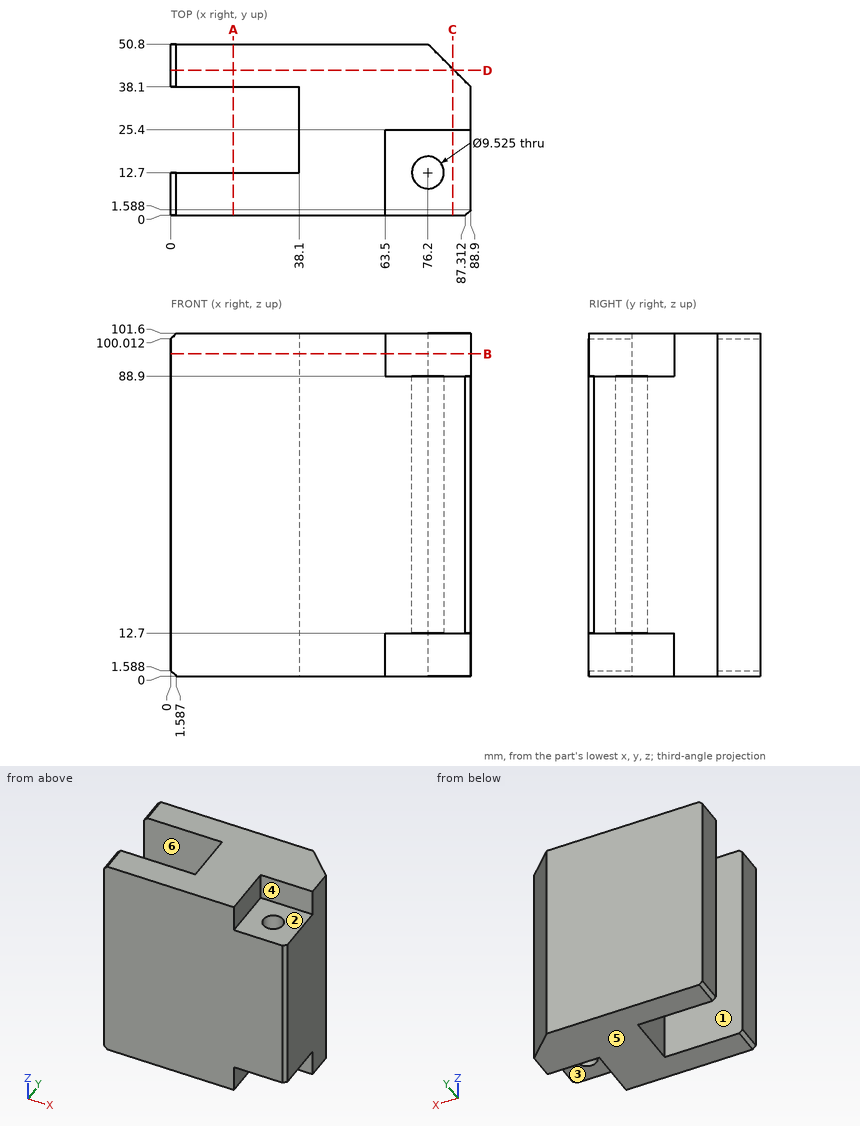
Here's the drawing with two shaded views (mm, measured from the low corner). I have some questions. A direction names the side the tool comes from. Coordinates: 2 decimals unless noted, no trailing zeros. Write each loop counter-clockwise with the first axis right and the second up, starting at its lowest first coordinate (ties: lowest second). Pieces come first, ordered by that corner, then holes.
Item 1: I want a section at B-B on z = 95.5. Write out the boundary of the cut face in (x, y), and give its area (3 significant figures).
Item 2: I want a section at A-A on x = 18.5. Write out the boundary of the cut face in (y, z), and give its area (3 significant figures).
Item 3: I want a section at C-C on x = 83.5. Write out the boundary of the cut face in (y, z).
Item 4: Will these pins go through, and if not, where does the flat tip stop? pin 1 (7.5 mm diameter, centred on x = 74.5, y = 7.5, fed in from +Z); pin 2 (8 mm diameter, centred on y = 15, z = 69, fed in from -X); pin 3 (11 mm diameter, centred on x = 76.2, y = 12.7, fed in from -Z); pin 4 (6.5 mm diameter, centred on x = 81, z = 95, fed in from -Y).
Item 5: If I drill on line 1 (Y direction, x = 26.5, z = 83); line 2 (Y direction, x = 76, z = 72); line 3 (X direction, y = 23, z = 27), over which ranges is the centre line in solid material (lowest first)?
Item 6: I want a section at D-D on y = 43. Write out the boundary of the cut face in (x, z).
Item 7: If we mould it in two halves opening along Y, with no side actions, what happens to the marked faces 4, 5 and 6? For each: +Y half, -Y half, draft (parallel to the pull), parting line (faces both ways), or undercut.
Item 8: On a 3-axis mill with a long thin cutter (end or side, diameter ignored), from which of +Z, -Z, +X, -X, +Y, -Y can I reach the whole of each face in a straight line? I mean the marked faces 1, 2 and 3. Say none if no direction works.
Findings below:
1. outline: (0, 0) - (63.5, 0) - (63.5, 25.4) - (88.9, 25.4) - (88.9, 38.1) - (76.2, 50.8) - (0, 50.8) - (0, 38.1) - (38.1, 38.1) - (38.1, 12.7) - (0, 12.7) - close
1. area: 2,820 mm2
2. outline: (0, 0) - (12.7, 0) - (12.7, 101.6) - (0, 101.6) - close; (38.1, 0) - (50.8, 0) - (50.8, 101.6) - (38.1, 101.6) - close
2. area: 2,580 mm2
3. outline: (0, 12.7) - (25.4, 12.7) - (25.4, 0) - (43.5, 0) - (43.5, 101.6) - (25.4, 101.6) - (25.4, 88.9) - (0, 88.9) - close
4. pin 1: stops at z = 88.9
4. pin 2: stops at x = 0
4. pin 3: stops at z = 12.7
4. pin 4: stops at y = 25.4
5. line 1: y = 0 to 12.7, 38.1 to 50.8
5. line 2: y = 0 to 7.94, 17.46 to 50.8
5. line 3: x = 38.1 to 88.9
6. outline: (0, 1.59) - (1.59, 0) - (84, 0) - (84, 101.6) - (1.59, 101.6) - (0, 100.01) - close
7. face 4: -Y half
7. face 5: draft
7. face 6: undercut
8. face 1: +Z, -Z, -X
8. face 2: +Z, +X, -Y
8. face 3: -Z, +X, -Y
